CAD build for the part. Positions are in the model's coordinates, mm. A direction names the side the tool comes from. Round coordinates to 2 decimals unless told otherwise and drop trailing zeros. Order: outer loops, then holes, each group sorted by start corner. A loop starts at its lowest first (then second) coordinate and runs counter-clockwise, first axis right, second up. Notation, with made-up numbers: M -19,2 L 25,2 A8 ccw 25,16 Z; hole C 2.5,21.25 d9. An arc over 180 degrees is marked long. Answer as a JSON object with one key per item and string values.
```python
from build123d import *

# Parameters (mm, degrees)
F0_W     = 32
F0_H     = 16
F1_DEPTH = 8
F2_R     = 2.5
F3_DEPTH = 2
F4_W     = 29.6
F4_H     = 13.6
F4_R     = 3.267
F5_DEPTH = 6.8
F6_R     = 2.6
F7_DEPTH = 6
F8_R     = 2.6
F9_DEPTH = 6


with BuildPart() as f1:
    # F0 (on Top) → F1 (new body)
    with BuildSketch(Plane.XY):
        Rectangle(F0_W, F0_H)
    extrude(amount=F1_DEPTH)

    # F2 (on face) → F3 (join)
    with BuildSketch(Plane.XY.offset(8)):
        with Locations((-12, 4)):
            Circle(F2_R)
        with Locations((-4, 4)):
            Circle(F2_R)
        with Locations((4, 4)):
            Circle(F2_R)
        with Locations((12, 4)):
            Circle(F2_R)
        with Locations((12, -4)):
            Circle(F2_R)
        with Locations((4, -4)):
            Circle(F2_R)
        with Locations((-4, -4)):
            Circle(F2_R)
        with Locations((-12, -4)):
            Circle(F2_R)
    extrude(amount=F3_DEPTH)

    # F4 (on face) → F5 (cut)
    with BuildSketch(Plane(origin=(0, 0, 0), x_dir=(1, 0, 0), z_dir=(0, 0, -1))):
        Rectangle(F4_W, F4_H)
        with Locations((-8, 0)):
            Circle(F4_R, mode=Mode.SUBTRACT)
        Circle(F4_R, mode=Mode.SUBTRACT)
        with Locations((8, 0)):
            Circle(F4_R, mode=Mode.SUBTRACT)
    extrude(amount=-F5_DEPTH, mode=Mode.SUBTRACT)

    # F6 (on face) → F7 (cut)
    with BuildSketch(Plane(origin=(0, 0, 0), x_dir=(1, 0, 0), z_dir=(0, 0, -1))):
        Circle(F6_R)
        with Locations((8, 0)):
            Circle(F6_R)
    extrude(amount=-F7_DEPTH, mode=Mode.SUBTRACT)

    # F8 (on face) → F9 (cut)
    with BuildSketch(Plane(origin=(0, 0, 0), x_dir=(1, 0, 0), z_dir=(0, 0, -1))):
        with Locations((-8, 0)):
            Circle(F8_R)
    extrude(amount=-F9_DEPTH, mode=Mode.SUBTRACT)


solid = f1.part
```
Item 1: Saw through at C-C on z = 9.25. List the corners of the cut face in (x, y), and give its area (3 significant figures).
Worked answers:
{"outline": "C -12,-4 d5; C -12,4 d5; C -4,-4 d5; C -4,4 d5; C 4,-4 d5; C 4,4 d5; C 12,-4 d5; C 12,4 d5", "area": "157 mm2"}
Item 2: Saw through at A-A on z = 5.5. List the corners of the cut face in (x, y).
Worked answers:
{"outline": "M -16,-8 L 16,-8 L 16,8 L -16,8 Z; C -8,0 d6.53; C 0,0 d6.53; C 8,0 d6.53; hole M -14.8,-6.8 L 14.8,-6.8 L 14.8,6.8 L -14.8,6.8 Z; hole C -8,0 d5.2; hole C 0,0 d5.2; hole C 8,0 d5.2"}
Item 3: Drop a flat-ended pin along its axis: pin 1 Ø1.6 at (x, y) = (-7.5, 0.5) entering from -Z. Give the stop position or say it passes through.
Worked answers:
{"pin 1": "stops at z = 6"}
Item 4: Saw through at D-D on x = -8. List the corners of the cut face in (y, z).
Worked answers:
{"outline": "M -8,0 L -6.8,0 L -6.8,6.8 L -3.27,6.8 L -3.27,0 L -2.6,0 L -2.6,6 L 2.6,6 L 2.6,0 L 3.27,0 L 3.27,6.8 L 6.8,6.8 L 6.8,0 L 8,0 L 8,8 L -8,8 Z"}
Item 5: Saw through at B-B on y = 4. List the corners of the cut face in (x, z), and give its area (3 significant figures).
Worked answers:
{"outline": "M -16,0 L -14.8,0 L -14.8,6.8 L 14.8,6.8 L 14.8,0 L 16,0 L 16,8 L 14.5,8 L 14.5,10 L 9.5,10 L 9.5,8 L 6.5,8 L 6.5,10 L 1.5,10 L 1.5,8 L -1.5,8 L -1.5,10 L -6.5,10 L -6.5,8 L -9.5,8 L -9.5,10 L -14.5,10 L -14.5,8 L -16,8 Z", "area": "94.7 mm2"}
Item 6: 3-axis set-ups, long thin cutter, end or side, ignore diameter. For faces 1 (the cylindrical face through (6.385, 4.751, 8.986)), 2 (the flat face through (8, -3, 0)), 3 (the flat face through (14.8, 0, 3)): which of +Z, -Z, +X, -X, +Y, -Y reach the whole face in a straight line?
Worked answers:
{"face 1": "+Z", "face 2": "-Z, +X, -X, +Y, -Y", "face 3": "-Z"}
Item 7: Two-plate mould, pull along X, no slides. Class faces 4 (the cylindrical face through (-0.338, -2.578, 2.958)), 5 (the flat face through (-1, -7, 0)): released by +X, released by -X, zero draft, split by the parting line, or undercut.
Worked answers:
{"face 4": "undercut", "face 5": "zero draft"}
Item 8: Wall check: line 1 along Y through (x, z) = (-8, 2.9); line 2 along Y through (x, z) = (-12.5, 2.25); line 3 along Y through (x, z) = (9.5, 2.5). Give the ranges that are in metal, low to high. Write a range as [from, to].
Worked answers:
{"line 1": "y = [-8, -6.8], [-3.27, -2.6], [2.6, 3.27], [6.8, 8]", "line 2": "y = [-8, -6.8], [6.8, 8]", "line 3": "y = [-8, -6.8], [-2.9, -2.12], [2.12, 2.9], [6.8, 8]"}
